from build123d import *

# Parameters (mm, degrees)
SKETCH_R        = 1.6
PAD_DEPTH       = 5
PAD001_DEPTH    = 7
COPYSKETCH002_W = 10
COPYSKETCH002_H = 18
POCKET_DEPTH    = 19.5
PAD002_DEPTH    = 3
POCKET001_DEPTH = 5
SKETCH004_W     = 14
SKETCH004_H     = 6
POCKET002_DEPTH = 5
FILLET_R        = 2
FILLET001_R     = 2


with BuildPart() as part:
    # Sketch → Pad (new body)
    with BuildSketch(Plane.XY):
        with BuildLine():
            Line((-25, 7.5), (25, 7.5))
            ThreePointArc((30, 2.5), (28.535534, 6.035534), (25, 7.5))
            Line((30, 2.5), (30, -2.5))
            ThreePointArc((25, -7.5), (28.535534, -6.035534), (30, -2.5))
            Line((25, -7.5), (-25, -7.5))
            ThreePointArc((-30, -2.5), (-28.535534, -6.035534), (-25, -7.5))
            Line((-30, -2.5), (-30, 2.5))
            ThreePointArc((-25, 7.5), (-28.535534, 6.035534), (-30, 2.5))
        make_face()
        with Locations((-25, 0)):
            Circle(SKETCH_R, mode=Mode.SUBTRACT)
        with Locations((25, 0)):
            Circle(SKETCH_R, mode=Mode.SUBTRACT)
    extrude(amount=PAD_DEPTH)

    # Sketch001 → Pad001 (join, symmetric)
    with BuildSketch(Plane.YZ):
        Polygon((-7.5, 5), (7.5, 5), (7.5, 0), (15, 8), (15, 23), (12, 23), align=None)
    extrude(amount=PAD001_DEPTH, both=True)

    # CopySketch002 → Pocket (cut)
    with BuildSketch(Plane.XZ.offset(7.5)):
        with Locations((0, 16)):
            Rectangle(COPYSKETCH002_W, COPYSKETCH002_H)
    extrude(amount=-POCKET_DEPTH, mode=Mode.SUBTRACT)

    # Sketch003 (on Face18 of Pocket) → Pad002 (join)
    with BuildSketch(Plane(origin=(0, 15, 0), x_dir=(-1, 0, 0), z_dir=(0, 1, 0))):
        with BuildLine():
            Line((-18, 23), (18, 23))
            ThreePointArc((21, 20), (20.12132, 22.12132), (18, 23))
            Line((21, 20), (21, 11))
            ThreePointArc((18, 8), (20.12132, 8.87868), (21, 11))
            Line((18, 8), (-18, 8))
            ThreePointArc((-21, 11), (-20.12132, 8.87868), (-18, 8))
            Line((-21, 11), (-21, 20))
            ThreePointArc((-18, 23), (-20.12132, 22.12132), (-21, 20))
        make_face()
        with BuildLine():
            Line((-18.5, 13.05), (-16.5, 13.05))
            ThreePointArc((-16.5, 10.95), (-15.45, 12), (-16.5, 13.05))
            Line((-18.5, 10.95), (-16.5, 10.95))
            ThreePointArc((-18.5, 13.05), (-19.55, 12), (-18.5, 10.95))
        make_face(mode=Mode.SUBTRACT)
        with BuildLine():
            Line((16.5, 13.05), (18.5, 13.05))
            ThreePointArc((18.5, 10.95), (19.549988, 12), (18.5, 13.05))
            Line((16.5, 10.95), (18.5, 10.95))
            ThreePointArc((16.5, 13.05), (15.45, 12), (16.5, 10.95))
        make_face(mode=Mode.SUBTRACT)
        with BuildLine():
            Line((-1.55, 16.999987), (-1.55, 13.999987))
            ThreePointArc((-1.55, 13.999987), (0, 12.45), (1.55, 13.999987))
            Line((1.55, 16.999987), (1.55, 13.999987))
            ThreePointArc((1.55, 16.999987), (0, 18.549987), (-1.55, 16.999987))
        make_face(mode=Mode.SUBTRACT)
    extrude(amount=-PAD002_DEPTH)

    # Pad002 Face28 → Pocket001 (cut)
    with BuildSketch(Plane(origin=(0, 15, 15.499993), x_dir=(1, 0, 0), z_dir=(0, 1, 0))):
        with BuildLine():
            ThreePointArc((-1.55, -1.499993), (0, -3.049993), (1.55, -1.499993))
            Line((1.55, -1.499993), (1.55, 1.500007))
            ThreePointArc((1.55, 1.500007), (0, 3.049993), (-1.55, 1.500007))
            Line((-1.55, 1.500007), (-1.55, -1.499993))
        make_face()
    extrude(amount=-POCKET001_DEPTH, mode=Mode.SUBTRACT)

    # Sketch004 (on Face18 of Pad002) → Pocket002 (cut)
    with BuildSketch(Plane(origin=(0, 15, 0), x_dir=(-1, 0, 0), z_dir=(0, 1, 0))):
        with Locations((-14, 20)):
            Rectangle(SKETCH004_W, SKETCH004_H)
        with Locations((14, 20)):
            Rectangle(SKETCH004_W, SKETCH004_H)
    extrude(amount=-POCKET002_DEPTH, mode=Mode.SUBTRACT)

    # Fillet
    fillet_edges = [part.edges().sort_by_distance(p)[0] for p in [
        (21, 13.5, 17),
    ]]
    fillet(fillet_edges, radius=FILLET_R)

    # Fillet001
    fillet001_edges = [part.edges().sort_by_distance(p)[0] for p in [
        (-21, 13.5, 17),
    ]]
    fillet(fillet001_edges, radius=FILLET001_R)


solid = part.part
Geometry: final body of the model. Coordinates: model frame, mm. A direction names the side the tool comes from. Round coordinates to 2 decimals unless told otherwise and drop trailing zeros. Loops run counter-clockwise (first coordinate to the right, second up) from the corner with the lowest first, then second, coordinate; pieces in that order, holes last.
Q1. Material intervals for L1, parallel to X at y = 11.5, z = 21.75; L2, parallel to Y at x = -25, z = 3.4; L3, parallel to Y at x = -21, z = 2.25, sorted ascending.
Q2. Pull-direction query (Z, two-part tool) for faces 5 (the flat face through (12, 14, 8)), 6 (the flat face through (-17, 14, 10.95)), 7 (the cylindrical face through (23.82, 1.08, 2.46)), 8 (the flat face through (-18, 0, 5)); classes: released by +Z, released by -Z, zero draft, split by the parting line, or undercut.
Q3. Section A-A on x = 0. Return loops of the section in (y, z), plus the area to 3 significant figures.
Q4. Section D-D on z = 18. Return loops of the section in (x, y), plus the area to 3 significant figures.
Q5. Section C-C on y = 0. Return loops of the section in (x, z), plus the area to 3 significant figures.
Q6. Pin query (flat end, axial travel): P1, Ø0.9, axis at y = 14, z = 15.5, coming from the +X side; P2, Ø1, axis at x = -3, z = 10, coming from the -Y side; P3, Ø1.6, axis at x = 17, y = 13.5, coming from the +Z side; P4, Ø1.9, axis at x = 25, y = 0, coming from the +Z side. Return the tip coordinate at first contact, or that it passes through.
Q7. Section B-B on z = 2.75. Return loops of the section in (x, y), plus the area to 3 significant figures.
Q8. Access query for faces 1 (the flat face through (2, 12, 15)), 2 (the flat face through (0, 14, 23)), 3 (the cylindrical face through (15.45, 13.52, 11.98)), 4 (the flat face through (19, 0, 5)). Directions: +Z, -Z, +X, -X, +Y, -Y. A direction counts if a zero-diameter tool reaches every point of the face in a straight line with its end or side. Return the directions, or none.
Evaluation:
1. L1: x = -7 to -5, 5 to 7
1. L2: y = -7.5 to -1.6, 1.6 to 7.5
1. L3: y = -7.5 to 7.5
2. face 5: released by -Z
2. face 6: undercut
2. face 7: zero draft
2. face 8: released by +Z
3. outline: (-7.5, 0) - (7.5, 0) - (15, 8) - (15, 12.45) - (12, 12.45) - (12, 7) - (-5.33, 7) - (-7.5, 5) - close; (12, 18.55) - (15, 18.55) - (15, 23) - (12, 23) - close
3. area: 155 mm2
4. outline: (-7, 6.58) - (-5, 6.58) - (-5, 12) - (-1.18, 12) - (-1.18, 15) - (-7, 15) - close; (1.18, 12) - (5, 12) - (5, 6.58) - (7, 6.58) - (7, 15) - (1.18, 15) - close
4. area: 56.6 mm2
5. outline: (-30, 0) - (-26.6, 0) - (-26.6, 5) - (-30, 5) - close; (-23.4, 0) - (23.4, 0) - (23.4, 5) - (7, 5) - (7, 11.92) - (5, 11.92) - (5, 7) - (-5, 7) - (-5, 11.92) - (-7, 11.92) - (-7, 5) - (-23.4, 5) - close; (26.6, 0) - (30, 0) - (30, 5) - (26.6, 5) - close
5. area: 316 mm2
6. P1: stops at x = 21
6. P2: stops at y = 12
6. P3: stops at z = 17
6. P4: passes through
7. outline: (-30, -2.5) arc R5 ccw to (-25, -7.5) - (25, -7.5) arc R5 ccw to (30, -2.5) - (30, 2.5) arc R5 ccw to (25, 7.5) - (7, 7.5) - (7, 10.08) - (-7, 10.08) - (-7, 7.5) - (-25, 7.5) arc R5 ccw to (-30, 2.5) - close; hole circle Ø3.2 at (-25, 0); hole circle Ø3.2 at (25, 0)
7. area: 899 mm2
8. face 1: +Z, -Y
8. face 2: +Z, +X, -X, +Y, -Y
8. face 3: +Y, -Y
8. face 4: +Z, +X, +Y, -Y
